Input: part model. Units: mm. Frame: model coordinates. A direction names the side the tool comes from. Coordinates: 2 decimals unless noted, no trailing zeros. Loops run counter-clockwise (first coordinate to the right, second up) from the corner with the lowest first, then second, coordinate; pieces in that order, holes last. Notation, with made-up numbers: M -5,42.25 L 18,42.25 A26 ccw 18,75.25 Z; hole C 78,-35.5 d7. An arc over 180 degrees is marked long. Use a Markdown table: item, result. Add a question column.
1. Section D-D on x = -31.5. Output: boundary loops of the cut face in (y, z), then the cut area to 3 significant figures.
2. Section C-C on y = -12. Output: boundary loops of the cut face in (x, z), then the cut area to 3 significant figures.
3. Draft query along X for faces 5 (the cylindrical face through (8.302, -17.998, 16.549)), 6 (the flat face through (-37.4, -19, 43.8)), 7 (the cylindrical face through (-76.148, -40.996, 9.86)), 8 (the flat face through (-45, 0, 7)). Return one class per face: +X half, -X half, draft (parallel to the pull), parting line (faces both ways), or undercut.
4. Set-up query: faces 1 (the flat face through (-75, -30, 25)), 2 (the flat face through (3.5, 0, 10)), 3 (the cylindrical face through (8.698, 17.998, 16.549)), 4 (the flat face through (-66.5, -22, 3)). Return all of +Z, -Z, +X, -X, +Y, -Y with unobstructed straight access to the full face (end or side cutting, diameter ignored); none if empty.
5. Line query: L1, parallel to Z at x = -31.5, y = -9; L2, parallel to Y at x = -76.5, z = 16.5; L3, parallel to X at y = 0, z = 24. Output: solid intervals per line, ascending. Write a range as [from, to].
6. Section B-B on x = 19. Output: boundary loops of the cut face in (y, z), then the cut area to 3 significant figures.
7. Pin query (flat end, axial travel): pin 1 (5 mm diameter, centred on x = -4.5, z = 31.5, fed in from +Y); pin 2 (4 mm diameter, centred on x = -79.5, y = -25.5, fed in from +Z); pin 3 (10 mm diameter, centred on x = -24, z = 24, fed in from -Y). Return the tip coordinate at first contact, or that it passes through.
8. Section A-A on y = 0. State how many separate pieces and enclosed holes the cut face has, then the cut area to 3 significant figures.
Autodesk Fusion 360 part; units mm, degrees
sketch "Sketch1" plane through (0, 0, 0) normal (0, 0, 1) x (1, 0, 0)
  line L0 (28.5, 25) -> (-60.5, 25)
  line L1 (-60.5, -25) -> (28.5, -25)
  line L2 (60.5, 25) -> (-60.5, -25) construction
  line L3 (-60.5, 25) -> (60.5, -25) construction
  line L4 (-92.5, 25) -> (-92.5, -25)
  arc A0 (-92.5, -25) -> (-60.5, -25) centre (-76.5, -25) ccw
  arc A1 (-60.5, 25) -> (-92.5, 25) centre (-76.5, 25) ccw
  line L5 (-76.5, 25) -> (-76.5, -25) construction
  line L6 (28.5, 25) -> (28.5, -25)
  line L7 (28.5, 25) -> (28.5, -25)
  line L8 (-60.5, 25) -> (28.5, 25)
  dimension "d1" = 121
  dimension "d2" = 50
  dimension "d3" = 16
  dimension "d4" = 32
  dimension "d5" = 121
extrude "Extrude1" add sketch "Sketch1" along normal blind 20
sketch "Sketch2" plane through (0, 0, 20) normal (0, 0, 1) x (-1, 0, 0)
  line L0 (92.5, -25) -> (92.5, 25)
  arc A0 (92.5, 25) -> (60.5, 25) centre (76.5, 25) ccw
  line L1 (60.5, 25) -> (-28.5, 25)
  line L2 (-28.5, 25) -> (-28.5, -25)
  line L3 (-28.5, -25) -> (60.5, -25)
  arc A1 (60.5, -25) -> (92.5, -25) centre (76.5, -25) ccw
  circle A2 centre (76.5, -25) radius 7
  circle A3 centre (76.5, 25) radius 7
  circle A4 centre (76.5, -25) radius 5
  circle A5 centre (76.5, 25) radius 5
  dimension "d8" = 14
  dimension "d9" = 14
  dimension "d10" = 10
  dimension "d11" = 10
extrude "Extrude2" cut sketch "Sketch2" against normal blind 45 contours A4 | A5
sketch "Sketch3" plane through (0, 0, 20) normal (0, 0, 1) x (-1, 0, 0)
  circle A0 centre (76.5, 25) radius 5
  circle A1 centre (76.5, -25) radius 5
  line L0 (92.5, -25) -> (92.5, 25)
  arc A2 (92.5, 25) -> (60.5, 25) centre (76.5, 25) ccw
  line L1 (60.5, 25) -> (-28.5, 25)
  line L2 (-28.5, 25) -> (-28.5, -25)
  line L3 (-28.5, -25) -> (60.5, -25)
  arc A3 (60.5, -25) -> (92.5, -25) centre (76.5, -25) ccw
  circle A4 centre (76.5, -25) radius 7
  circle A5 centre (76.5, 25) radius 7
  dimension "d14" = 14
  dimension "d15" = 14
extrude "Extrude3" add sketch "Sketch3" along normal blind 5 contours A4 | A5
sketch "Sketch4" plane through (0, 0, 0) normal (0, 0, -1) x (1, 0, 0)
  circle A0 centre (-76.5, 25) radius 5
  circle A1 centre (-76.5, -25) radius 5
  line L0 (-92.5, 25) -> (-92.5, -25)
  arc A2 (-92.5, -25) -> (-60.5, -25) centre (-76.5, -25) ccw
  line L1 (-60.5, -25) -> (28.5, -25)
  line L2 (28.5, -25) -> (28.5, 25)
  line L3 (28.5, 25) -> (-60.5, 25)
  arc A3 (-60.5, 25) -> (-92.5, 25) centre (-76.5, 25) ccw
  line L4 (-86.5, 25) -> (-86.5, -25)
  arc A4 (-86.5, -25) -> (-66.5, -25) centre (-76.5, -25) ccw
  arc A5 (-66.5, 25) -> (-86.5, 25) centre (-76.5, 25) ccw
  line L5 (-76.5, 25) -> (-76.5, -25) construction
  line L6 (-30, 25) -> (-30, 19) construction
  line L7 (28.5, 0) -> (22.5, 0) construction
  line L8 (22.5, 19) -> (22.5, 0)
  line L9 (22.5, 19) -> (-66.5, 19)
  line L10 (22.5, 0) -> (22.5, -19)
  line L11 (22.5, -19) -> (-66.5, -19)
  line L12 (-66.5, -25) -> (-66.5, -19)
  line L13 (-66.5, 19) -> (-66.5, 25)
  dimension "d18" = 20
  dimension "d19" = 6
  dimension "d20" = 6
  dimension "d21" = 19
extrude "Extrude4" cut sketch "Sketch4" against normal blind 7 contours L4 A4 A5 L8 L9 L10 L11 L12 L13
sketch "Sketch5" plane through (0, 0, 20) normal (0, 0, 1) x (-1, 0, 0)
  circle A0 centre (76.5, 25) radius 7
  circle A1 centre (76.5, -25) radius 7
  line L0 (92.5, -25) -> (92.5, 25)
  arc A2 (92.5, 25) -> (60.5, 25) centre (76.5, 25) ccw
  line L1 (60.5, 25) -> (-28.5, 25)
  line L2 (-28.5, 25) -> (-28.5, -25)
  line L3 (-28.5, -25) -> (60.5, -25)
  arc A3 (60.5, -25) -> (92.5, -25) centre (76.5, -25) ccw
  line L4 (-28.5, 0) -> (-28.5, -9)
  line L5 (-28.5, 0) -> (-28.5, 9)
  line L6 (-28.5, -25) -> (-8.5, -25)
  line L7 (-8.5, -9) -> (-8.5, 9)
  line L8 (0.5, -9) -> (0.5, 9)
  arc A4 (0.5, 9) -> (-17.5, 9) centre (-8.5, 9) ccw
  line L9 (-17.5, 9) -> (-17.5, -9)
  arc A5 (-17.5, -9) -> (0.5, -9) centre (-8.5, -9) ccw
  line L10 (-8.5, -9) -> (-8.5, 9) construction
  line L11 (-3.5, -9) -> (-3.5, 9)
  arc A6 (-3.5, 9) -> (-13.5, 9) centre (-8.5, 9) ccw
  line L12 (-13.5, 9) -> (-13.5, -9)
  arc A7 (-13.5, -9) -> (-3.5, -9) centre (-8.5, -9) ccw
  line L13 (-8.5, -9) -> (-8.5, 9) construction
  dimension "d24" = 9
  dimension "d25" = 9
  dimension "d26" = 20
  dimension "d27" = 18
  dimension "d28" = 10
extrude "Extrude5" cut sketch "Sketch5" against normal blind 7 contours L8 A4 L9 A5
extrude "Extrude6" cut 1 faces at (10.1667, -3, 20) along direction (0, 0, -1) blind 55
sketch "Sketch6" plane through (0, 0, 20) normal (0, 0, 1) x (-1, 0, 0)
  line L0 (92.5, -25) -> (92.5, 25)
  arc A0 (92.5, 25) -> (60.5, 25) centre (76.5, 25) ccw
  line L1 (60.5, 25) -> (-28.5, 25)
  line L2 (-28.5, 25) -> (-28.5, -25)
  line L3 (-28.5, -25) -> (60.5, -25)
  arc A1 (60.5, -25) -> (92.5, -25) centre (76.5, -25) ccw
  circle A2 centre (76.5, -25) radius 7
  circle A3 centre (76.5, 25) radius 7
  line L4 (0.5, 9) -> (0.5, -9)
  arc A4 (-17.5, -9) -> (0.5, -9) centre (-8.5, -9) ccw
  line L5 (-17.5, -9) -> (-17.5, 9)
  arc A5 (0.5, 9) -> (-17.5, 9) centre (-8.5, 9) ccw
sketch "Sketch7" plane through (0, 0, 20) normal (0, 0, 1) x (-1, 0, 0)
  line L0 (-28.5, -25) -> (31.5, -25)
  dimension "d33" = 60
sketch "Sketch8" plane through (0, 0, 20) normal (0, 0, 1) x (-1, 0, 0)
  line L0 (31.5, -25) -> (31.5, 0)
  arc A0 (-13.5, -9) -> (-3.5, -9) centre (-8.5, -9) ccw
  line L1 (-3.5, -9) -> (-3.5, 9)
  arc A1 (-3.5, 9) -> (-13.5, 9) centre (-8.5, 9) ccw
  line L2 (-13.5, 9) -> (-13.5, -9)
  circle A2 centre (76.5, 25) radius 5
  circle A3 centre (76.5, -25) radius 5
  line L3 (-22.5, 19) -> (66.5, 19)
  line L4 (66.5, 19) -> (66.5, 25)
  arc A4 (86.5, 25) -> (66.5, 25) centre (76.5, 25) ccw
  line L5 (86.5, 25) -> (86.5, -25)
  arc A5 (66.5, -25) -> (86.5, -25) centre (76.5, -25) ccw
  line L6 (66.5, -25) -> (66.5, -19)
  line L7 (66.5, -19) -> (-22.5, -19)
  line L8 (-22.5, -19) -> (-22.5, 19)
  line L9 (31.5, -19) -> (56.5, -19)
  line L10 (31.5, 19) -> (6.5, 19)
  line L11 (6.5, 19) -> (56.5, 19)
  line L12 (56.5, 19) -> (56.5, -19)
  line L13 (56.5, -19) -> (6.5, -19)
  line L14 (6.5, -19) -> (6.5, 19)
  dimension "d34" = 25
  dimension "d35" = 25
extrude "Extrude7" add sketch "Sketch8" along normal blind 35 contours L3 L7 L9 L10 L11 L12 L13 L14
sketch "Sketch9" plane through (0, -19, 0) normal (0, -1, 0) x (1, 0, 0)
  line L0 (-56.5, 20) -> (-6.5, 20)
  line L1 (-6.5, 20) -> (-6.5, 55)
  line L2 (-6.5, 55) -> (-56.5, 55)
  line L3 (-56.5, 55) -> (-56.5, 20)
  circle A0 centre (-31.5, 55) radius 25
  dimension "d38" = 50
extrude "Extrude8" add sketch "Sketch9" against normal blind 38 contours L2 A0 picked at (-35.1673, 71.0673)
sketch "Sketch10" plane through (0, -19, 0) normal (0, -1, 0) x (1, 0, 0)
  line L0 (-56.5, 20) -> (-6.5, 20)
  line L1 (-6.5, 20) -> (-6.5, 55)
  arc A0 (-6.5, 55) -> (-56.5, 55) centre (-31.5, 55) ccw
  line L2 (-56.5, 55) -> (-56.5, 20)
  circle A1 centre (-31.5, 55) radius 12.5
  dimension "d41" = 25
extrude "Extrude9" cut sketch "Sketch10" against normal blind 70 contours A1
sketch "Sketch11" plane through (0, 0, 7) normal (0, 0, -1) x (1, 0, 0)
  arc A0 (3.5, -9) -> (13.5, -9) centre (8.5, -9) ccw
  line L0 (3.5, -9) -> (3.5, 9)
  arc A1 (13.5, 9) -> (3.5, 9) centre (8.5, 9) ccw
  line L1 (13.5, 9) -> (13.5, -9)
  circle A2 centre (-76.5, 25) radius 5
  circle A3 centre (-76.5, -25) radius 5
  line L2 (22.5, 19) -> (-66.5, 19)
  line L3 (-66.5, 19) -> (-66.5, 25)
  arc A4 (-66.5, 25) -> (-86.5, 25) centre (-76.5, 25) ccw
  line L4 (-86.5, 25) -> (-86.5, -25)
  arc A5 (-86.5, -25) -> (-66.5, -25) centre (-76.5, -25) ccw
  line L5 (-66.5, -25) -> (-66.5, -19)
  line L6 (-66.5, -19) -> (22.5, -19)
  line L7 (22.5, -19) -> (22.5, 19)
  line L8 (-66.5, 25) -> (-66.5, 19)
  line L9 (-66.5, 19) -> (22.5, 19)
  line L10 (22.5, 19) -> (22.5, -19)
  line L11 (22.5, -19) -> (-66.5, -19)
  line L12 (-66.5, -19) -> (-66.5, -25)
  arc A6 (-86.5, -25) -> (-66.5, -25) centre (-76.5, -25) ccw
  line L13 (-86.5, -25) -> (-86.5, 25)
  arc A7 (-66.5, 25) -> (-86.5, 25) centre (-76.5, 25) ccw
  line L14 (-92.5, 25) -> (-92.5, -25)
  arc A8 (-92.5, -25) -> (-60.5, -25) centre (-76.5, -25) ccw
  line L15 (-60.5, -25) -> (28.5, -25)
  line L16 (28.5, -25) -> (28.5, 25)
  line L17 (28.5, 25) -> (-60.5, 25)
  arc A9 (-60.5, 25) -> (-92.5, 25) centre (-76.5, 25) ccw
  line L18 (-92.5, 0) -> (-32, 0)
  circle A10 centre (-32, 0) radius 7
  dimension "d44" = 60.5
  dimension "d45" = 14
extrude "Extrude10" cut sketch "Sketch11" against normal blind 8 contours A10
sketch "Sketch12" plane through (0, 0, 15) normal (0, 0, -1) x (1, 0, 0)
  circle A0 centre (-32, 0) radius 7
  circle A1 centre (-32, 0) radius 15
  dimension "d48" = 30
extrude "Extrude11" cut sketch "Sketch12" against normal blind 15
extrude "Extrude12" cut 1 faces at (-31.572, 1.6695, 15) along direction (0, 0, 1) blind 15
equation "d2 = 0 mm + 50 mm"
equation "d44 = ( 121 / 2 ) * 1 mm"
Answers below:
| question | item | result |
|---|---|---|
| 1 | outline | M -25,0 L -19,0 L -19,7 L -6.98,7 L -6.98,15 L -14.99,15 L -14.99,30 L 14.99,30 L 14.99,15 L 6.98,15 L 6.98,7 L 19,7 L 19,0 L 25,0 L 25,20 L 19,20 L 19,42.5 L -19,42.5 L -19,20 L -25,20 Z; M -19,67.5 L 19,67.5 L 19,80 L -19,80 Z |
| 1 | area | 1,500 mm² |
| 2 | outline | M -92.5,0 L -86.5,0 L -86.5,7 L 4.5,7 L 4.5,13 L 0.01,13 L 0.01,20 L -6.5,20 L -6.5,55 A25 ccw -56.5,55 L -56.5,20 L -92.5,20 Z; M 12.5,7 L 22.5,7 L 22.5,0 L 28.5,0 L 28.5,20 L 16.99,20 L 16.99,13 L 12.5,13 Z; hole C -31.5,55 d25; hole M -41,15 L -23,15 L -23,30 L -41,30 Z |
| 2 | area | 3,460 mm² |
| 3 | face 5 | undercut |
| 3 | face 6 | draft |
| 3 | face 7 | parting line |
| 3 | face 8 | undercut |
| 4 | face 1 | +Z, -X, +Y, -Y |
| 4 | face 2 | +Z, -Z |
| 4 | face 3 | +Z |
| 4 | face 4 | -Z |
| 5 | L1 | z = [7, 15], [30, 42.5], [67.5, 80] |
| 5 | L2 | y = [-41, -30], [-20, 20], [30, 41] |
| 5 | L3 | x = [-56.5, -47], [-17, -6.5] |
| 6 | outline | M -25,0 L -19,0 L -19,7 L 19,7 L 19,0 L 25,0 L 25,20 L -25,20 Z |
| 6 | area | 734 mm² |
| 7 | pin 1 | stops at y = 19 |
| 7 | pin 2 | stops at z = 25 |
| 7 | pin 3 | stops at y = -25 |
| 8 | separate pieces | 2 |
| 8 | enclosed holes | 1 |
| 8 | area | 3,150 mm² |
